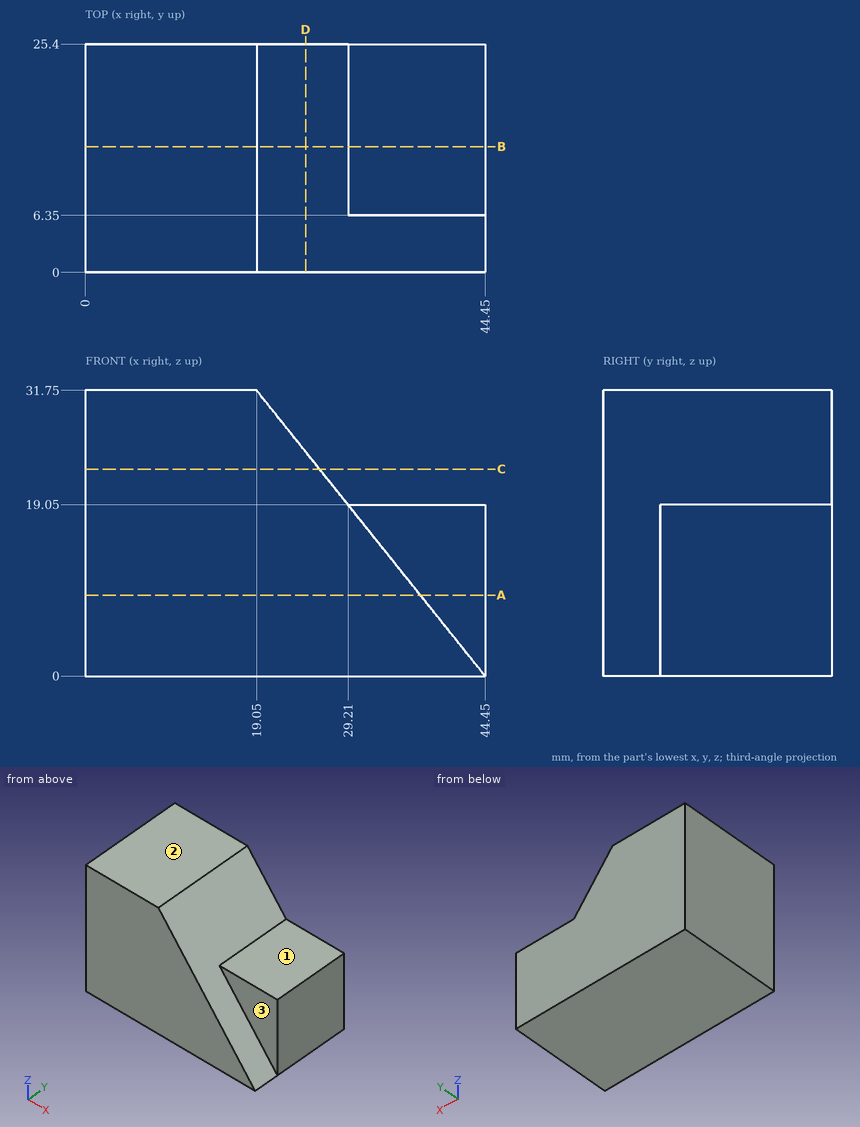
Geometry check sheet. Reference: drawing and pictorial views, mm from the part's lowest x, y, z. A direction names the side the tool comes from. Give positions to 0.01 mm unless a question says otherwise; leave off trailing zeros. Loops run counter-clockwise (first coordinate to the right, second up) from the corner with the lowest first, then second, coordinate; pieces in that order, holes last. Notation, with made-up numbers: (-17, 14.5) - (8, 14.5) arc R16 cw to (8, 45.5) - close; hole circle Ø4 at (-13.75, -37). An arc over 180 degrees is marked (long way). One line per question, with ' | ' between items. Start each with the question number.
1. Cross-section at A-A, the plane z = 9. Enter the section's corners in (x, y), plus the area to 3 significant figures.
2. Set-up check for the marked faces 1, 2 and 3: record each of +Z, -Z, +X, -X, +Y, -Y from which the full face is reachable in a straight line by a thin tool's end or side.
3. Cross-section at C-C, the plane z = 23. Enter the section's corners in (x, y).
4. Cross-section at D-D, the plane x = 24.5. Enter the section's corners in (y, z), plus the area to 3 significant figures.
5. Gauge pin test, flat ends, axial feed: pin 1 Ø2 at (x, y) = (36.5, 19.5) entering from +Z; pin 2 Ø12 at (x, y) = (34, 15.5) entering from +Z; pin 3 Ø5 at (y, z) = (2.5, 8.5) entering from +X. Record the tip position at first contact, or that the pin passes through.
6. Material ranges on line 1 along Z through (x, y) = (34, 21); line 2 along Y through (x, z) = (34.5, 17); line 3 along X through (y, z) = (2, 25), recorded low to high. Write a range as [from, to].
7. Cross-section at B-B, the plane y = 14. Enter the section's corners in (x, z), plus the area to 3 significant figures.
Check result:
1) outline: (0, 0) - (37.25, 0) - (37.25, 6.35) - (44.45, 6.35) - (44.45, 25.4) - (0, 25.4) - close | area: 1,080 mm2
2) face 1: +Z, +X, +Y, -Y | face 2: +Z, +X, -X, +Y, -Y | face 3: +Z, +X, -Y
3) outline: (0, 0) - (26.05, 0) - (26.05, 25.4) - (0, 25.4) - close
4) outline: (0, 0) - (25.4, 0) - (25.4, 24.94) - (0, 24.94) - close | area: 633 mm2
5) pin 1: stops at z = 19.05 | pin 2: stops at z = 20.56 | pin 3: stops at x = 39.65
6) line 1: z = [0, 19.05] | line 2: y = [6.35, 25.4] | line 3: x = [0, 24.45]
7) outline: (0, 0) - (44.45, 0) - (44.45, 19.05) - (29.21, 19.05) - (19.05, 31.75) - (0, 31.75) - close | area: 1,150 mm2
